Source: CAD feature listing. Evaluate the final solid. Frame: model axes, mm. Face numbers are marked on the shaded views. A direction names the side the tool comes from. Give positions to 0.01 mm unless a question says otherwise; leave off trailing zeros. Order: outer loops, then holes, each group sorted by start corner. A loop starts at its lowest first (then second) coordinate and runs counter-clockwise, first axis right, second up. Notation, with made-up numbers: (-17.75, -21.5) -> (16.25, -21.5) arc R10 cw to (16.25, -9.5) -> close; hole circle Ø3 at (64, 51.25). An arc over 180 degrees is marked (long way). Use one line per item in the form item = value. Start each with the question number.
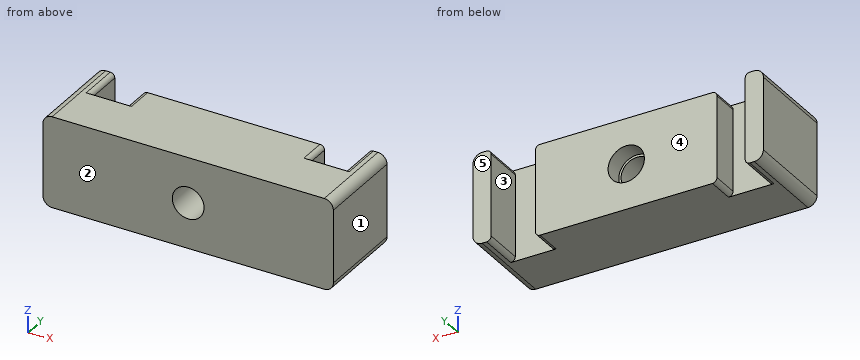
from build123d import *

# Parameters (mm, degrees)
BOSS_EXTRUDE1_DEPTH = 10
SKETCH2_R           = 1.75
CUT_EXTRUDE1_DEPTH  = 22.354156504
FILLET2_R           = 1
FILLET3_R           = 0.5
SKETCH4_W           = 20
SKETCH4_H           = 10
CUT_EXTRUDE3_DEPTH  = 1.5
SKETCH5_R           = 2
CUT_EXTRUDE4_DEPTH  = 2


with BuildPart() as part:
    # Sketch1 → Boss-Extrude1 (new body)
    with BuildSketch(Plane.XY):
        Polygon((-10, 2.5), (10, 2.5), (10, 0), (10, -2), (14, -2), (14, 0), (14, 2.5), (16, 2.5), (16, -7.5), (-16, -7.5), (-16, 2.5), (-14, 2.5), (-14, 0), (-14, -2), (-10, -2), (-10, 0), align=None)
    extrude(amount=BOSS_EXTRUDE1_DEPTH)

    # Sketch2 → Cut-Extrude1 (cut, through all)
    with BuildSketch(Plane(origin=(0, 2.5, 0), x_dir=(1, 0, 0), z_dir=(0, 1, 0))):
        with Locations(Location((0, -5, 0), (0, 0, 270))):
            Circle(SKETCH2_R)
    extrude(amount=-CUT_EXTRUDE1_DEPTH, mode=Mode.SUBTRACT)

    # Fillet2
    fillet2_edges = [part.edges().sort_by_distance(p)[0] for p in [
        (16, -2.5, 0),
        (-16, -2.5, 0),
        (-16, -2.5, 10),
        (16, -2.5, 10),
    ]]
    fillet(fillet2_edges, radius=FILLET2_R)

    # Fillet3
    fillet3_edges = [part.edges().sort_by_distance(p)[0] for p in [
        (-10, 0.25, 10),
        (14, 0.25, 0),
        (-14, 0.25, 0),
        (-10, 0.25, 0),
        (10, 0.25, 0),
        (-14, 0.25, 10),
        (10, 0.25, 10),
        (14, 0.25, 10),
    ]]
    fillet(fillet3_edges, radius=FILLET3_R)

    # Sketch4 → Cut-Extrude3 (cut)
    with BuildSketch(Plane(origin=(0, 2.5, 0), x_dir=(1, 0, 0), z_dir=(0, 1, 0))):
        with Locations((0, -5)):
            Rectangle(SKETCH4_W, SKETCH4_H)
    extrude(amount=-CUT_EXTRUDE3_DEPTH, mode=Mode.SUBTRACT)

    # Sketch5 → Cut-Extrude4 (cut)
    with BuildSketch(Plane(origin=(0, 1, 0), x_dir=(1, 0, 0), z_dir=(0, 1, 0))):
        with Locations(Location((0, -5, 0), (0, 0, 270))):
            Circle(SKETCH5_R)
    extrude(amount=-CUT_EXTRUDE4_DEPTH, mode=Mode.SUBTRACT)


solid = part.part
1) Cut plane A-A, the plane y = 0. Return the cut outline in (x, z), plus the area to 3 significant figures.
2) Material intervals for probe 1 along X at (y, z) = (0.3, 5); probe 2 along X at (y, z) = (0.5, 1.75); probe 3 along X at (y, z) = (1.75, 6), sorted ascending.
3) Pin query (flat end, axial travel): pin 1 (1.5 mm diameter, centred on x = 12, z = 3, fed in from +Y); pin 2 (1.5 mm diameter, centred on x = -2, z = 8, fed in from +Y). Return the tip coordinate at first contact, or that it passes through.
4) Cut plane C-C, the plane y = 1.75. Return the cut outline in (x, z), plus the area to 3 significant figures.
5) Reachability of the marked faces 4 and 5 from +Z, -Z, +X, -X, +Y, -Y: full face, straight path, thin tool, end or side. Return the list, or none.
6) Cut plane D-D, the plane x = 0. Return the cut outline in (y, z), plus the area to 4 significant figures.
7) Cut plane B-B, the plane z = 5. Return the cut outline in (x, y).
8) Draft query along X for the marked faces 1, 2 and 3. Return one class per face: +X half, -X half, draft (parallel to the pull), parting line (faces both ways), or undercut.
Output values:
q1.outline = (-16, 1) arc R1 ccw to (-15, 0) -> (-14.5, 0) arc R0.5 ccw to (-14, 0.5) -> (-14, 9.5) arc R0.5 ccw to (-14.5, 10) -> (-15, 10) arc R1 ccw to (-16, 9) -> close; (-10, 0.5) arc R0.5 ccw to (-9.5, 0) -> (9.5, 0) arc R0.5 ccw to (10, 0.5) -> (10, 9.5) arc R0.5 ccw to (9.5, 10) -> (-9.5, 10) arc R0.5 ccw to (-10, 9.5) -> close; (14, 0.5) arc R0.5 ccw to (14.5, 0) -> (15, 0) arc R1 ccw to (16, 1) -> (16, 9) arc R1 ccw to (15, 10) -> (14.5, 10) arc R0.5 ccw to (14, 9.5) -> close; hole circle Ø4 at (0, 5)
q1.area = 226 mm^2
q2.probe_1 = -16 to -14, -10 to -2, 2 to 10, 14 to 16
q2.probe_2 = -16 to -14, -10 to 10, 14 to 16
q2.probe_3 = -16 to -14, 14 to 16
q3.pin_1 = -2
q3.pin_2 = 1
q4.outline = (-16, 1) arc R1 ccw to (-15, 0) -> (-14.5, 0) arc R0.5 ccw to (-14, 0.5) -> (-14, 9.5) arc R0.5 ccw to (-14.5, 10) -> (-15, 10) arc R1 ccw to (-16, 9) -> close; (14, 0.5) arc R0.5 ccw to (14.5, 0) -> (15, 0) arc R1 ccw to (16, 1) -> (16, 9) arc R1 ccw to (15, 10) -> (14.5, 10) arc R0.5 ccw to (14, 9.5) -> close
q4.area = 38.9 mm^2
q5.face_4 = +Z, -Z, +Y
q5.face_5 = +Z, -Z, +X, -X, +Y
q6.outline = (-7.5, 0) -> (1, 0) -> (1, 3) -> (-1, 3) -> (-1, 3.25) -> (-7.5, 3.25) -> close; (-7.5, 6.75) -> (-1, 6.75) -> (-1, 7) -> (1, 7) -> (1, 10) -> (-7.5, 10) -> close
q6.area = 54.25 mm^2
q7.outline = (-16, -7.5) -> (-1.75, -7.5) -> (-1.75, -1) -> (-2, -1) -> (-2, 1) -> (-10, 1) -> (-10, -2) -> (-14, -2) -> (-14, 2.5) -> (-16, 2.5) -> close; (1.75, -7.5) -> (16, -7.5) -> (16, 2.5) -> (14, 2.5) -> (14, -2) -> (10, -2) -> (10, 1) -> (2, 1) -> (2, -1) -> (1.75, -1) -> close
q8.face_1 = +X half
q8.face_2 = draft
q8.face_3 = undercut
